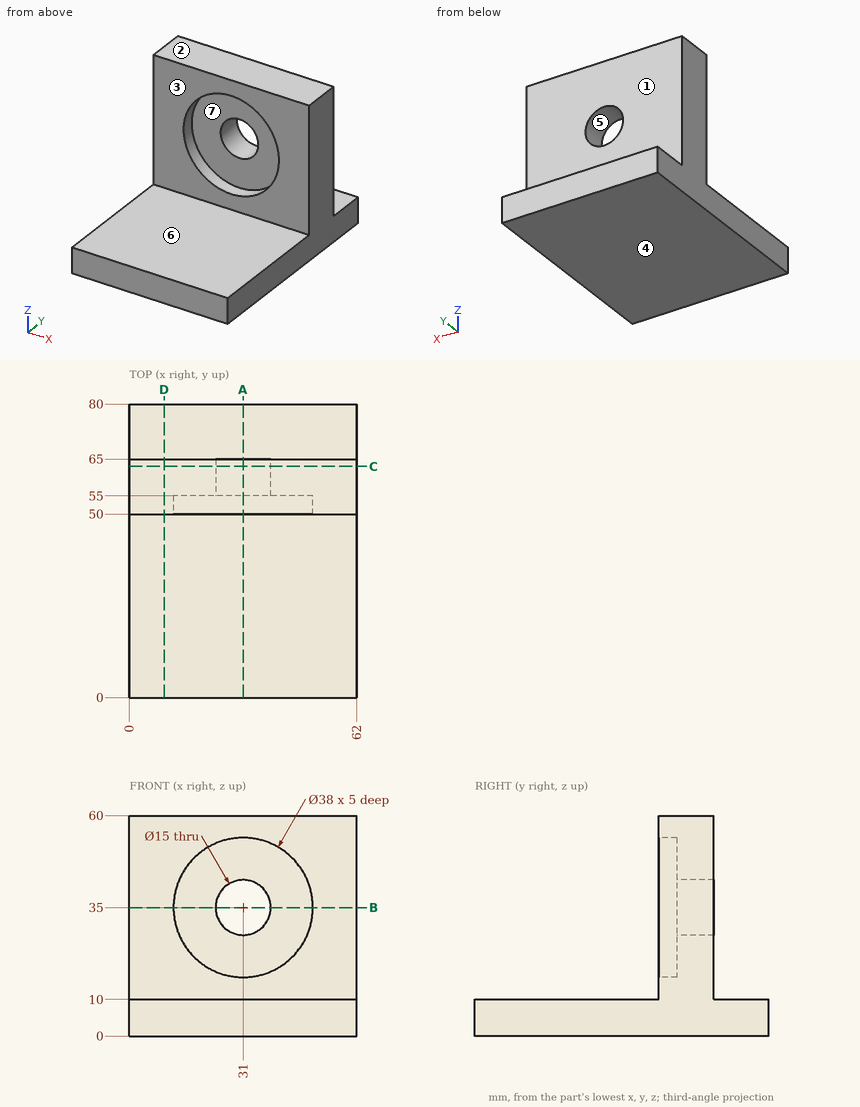
Print and shaded views of the part. All mm, measured from the part's lowest x, y and z. A direction names the side the tool comes from. Give positions to 0.01 mm unless a question says otherwise; leave off trailing zeros. Loops run counter-clockwise (first coordinate to the right, second up) from the corner with the lowest first, then second, coordinate; pieces in that order, holes last. Notation, with made-up numbers: (60.25, -7) - (101.25, -7) arc R20 ccw to (101.25, -1) - close; hole circle Ø10 at (-11.5, 56.5). An arc over 180 degrees is marked (long way). Use a Markdown table: item, result.
(1) Band-saw the part on D-D (x = 9.5). Give the cut face in (y, z), and give its area (3 significant figures).
Taken from the geometry:
| item | result |
|---|---|
| outline | (0, 0) - (80, 0) - (80, 10) - (65, 10) - (65, 60) - (50, 60) - (50, 10) - (0, 10) - close |
| area | 1,550 mm2 |
(2) Which spindle directions (+Z, -Z, +X, -X, +Y, -Y) get a long thin tool onto all of the face, cutting with end or side? Do the marked faces 1, 2 and 3. Say none if no direction does.
Taken from the geometry:
| item | result |
|---|---|
| face 1 | +Z, +X, -X, +Y |
| face 2 | +Z, +X, -X, +Y, -Y |
| face 3 | +Z, +X, -X, -Y |
(3) Band-saw the part on A-A (x = 31). Give the cut face in (y, z).
Taken from the geometry:
| item | result |
|---|---|
| outline | (0, 0) - (80, 0) - (80, 10) - (65, 10) - (65, 27.5) - (55, 27.5) - (55, 16) - (50, 16) - (50, 10) - (0, 10) - close; (50, 54) - (55, 54) - (55, 42.5) - (65, 42.5) - (65, 60) - (50, 60) - close |
(4) Drop flat-ended pins along their axis: pin 1 Ø10 at (x, z) = (14.5, 27) entering from -Y; pin 2 Ø16.5 at (x, y) = (21, 74) entering from +Z; pin 3 Ø6 at (x, z) = (51, 20) entering from +Y; pin 4 Ø1 at (x, y) = (13, 39) entering from -Z. Give the stop position or say it passes through.
Taken from the geometry:
| item | result |
|---|---|
| pin 1 | y = 50 |
| pin 2 | z = 10 |
| pin 3 | y = 65 |
| pin 4 | z = 0 |
(5) Band-saw the part on B-B (z = 35). Give the cut face in (x, y), and give its area (3 significant figures).
Taken from the geometry:
| item | result |
|---|---|
| outline | (0, 50) - (12, 50) - (12, 55) - (23.5, 55) - (23.5, 65) - (0, 65) - close; (38.5, 55) - (50, 55) - (50, 50) - (62, 50) - (62, 65) - (38.5, 65) - close |
| area | 590 mm2 |
(6) Wall check: line 1 along Z through (x, y) = (31, 51.9); line 2 along Z through (x, y) = (31, 59); line 3 along Z through (x, y) = (47.5, 17). Give the ranges that are in metal, low to high.
Taken from the geometry:
| item | result |
|---|---|
| line 1 | 0 to 16, 54 to 60 |
| line 2 | 0 to 27.5, 42.5 to 60 |
| line 3 | 0 to 10 |
(7) Band-saw the part on C-C (y = 63). Give the cut face in (x, z), and give its area (3 significant figures).
Taken from the geometry:
| item | result |
|---|---|
| outline | (0, 0) - (62, 0) - (62, 60) - (0, 60) - close; hole circle Ø15 at (31, 35) |
| area | 3,540 mm2 |
(8) Pull direction Z, two halves, no side cores. Call the marked faces 4, 5, 6 and 7: +Z half, -Z half, draft (parallel to the pull), parting line (faces both ways), or undercut.
Taken from the geometry:
| item | result |
|---|---|
| face 4 | -Z half |
| face 5 | undercut |
| face 6 | +Z half |
| face 7 | undercut |
